```python
from build123d import *

# Parameters (mm, degrees)
BOSS_EXTRUDE1_DEPTH = 4
SKETCH3_R           = 4
SKETCH3_R_2         = 1.5
CUT_EXTRUDE1_DEPTH  = 119.072218241
SKETCH5_R           = 1.5
CUT_EXTRUDE2_DEPTH  = 119.072218241
SKETCH6_R           = 1.5
CUT_EXTRUDE3_DEPTH  = 119.072218241


with BuildPart() as part:
    # Sketch1 → Boss-Extrude1 (new body)
    with BuildSketch(Plane(origin=(0, 0, 0), x_dir=(1, 0, 0), z_dir=(0, 1, 0))):
        Polygon((-55, 61.024984395), (-35, 42), (35, 42), (55, 61.024984395), (81, 61.024984395), (101, 40), (101, -40), (81, -61.024984395), (55, -61.024984395), (35, -42), (-35, -42), (-55, -61.024984395), (-81, -61.024984395), (-101, -40), (-101, 40), (-81, 61.024984395), align=None)
    extrude(amount=BOSS_EXTRUDE1_DEPTH)

    # Sketch3 → Cut-Extrude1 (cut, through all)
    with BuildSketch(Plane(origin=(0, 4, 0), x_dir=(1, 0, 0), z_dir=(0, 1, 0))):
        with Locations(Location((-35, -29, 0), (0, 0, 270))):
            Circle(SKETCH3_R)
        with Locations(Location((-28.5, -29, 0), (0, 0, 270))):
            Circle(SKETCH3_R_2)
        with Locations(Location((-41.5, -29, 0), (0, 0, 270))):
            Circle(SKETCH3_R_2)
        with Locations(Location((-35, -22.5, 0), (0, 0, 270))):
            Circle(SKETCH3_R_2)
        with Locations(Location((-35, -35.5, 0), (0, 0, 270))):
            Circle(SKETCH3_R_2)
        with Locations(Location((-35, 35.5, 0), (0, 0, 90))):
            Circle(SKETCH3_R_2)
        with Locations(Location((-35, 22.5, 0), (0, 0, 90))):
            Circle(SKETCH3_R_2)
        with Locations(Location((-41.5, 29, 0), (0, 0, 90))):
            Circle(SKETCH3_R_2)
        with Locations(Location((-28.5, 29, 0), (0, 0, 90))):
            Circle(SKETCH3_R_2)
        with Locations(Location((-35, 29, 0), (0, 0, 90))):
            Circle(SKETCH3_R)
        with Locations(Location((-35, 0, 0), (0, 0, 270))):
            Circle(SKETCH3_R)
        with Locations(Location((-35, 6.5, 0), (0, 0, 270))):
            Circle(SKETCH3_R_2)
        with Locations(Location((-28.5, 0, 0), (0, 0, 270))):
            Circle(SKETCH3_R_2)
        with Locations(Location((-41.5, 0, 0), (0, 0, 270))):
            Circle(SKETCH3_R_2)
        with Locations(Location((-35, -6.5, 0), (0, 0, 270))):
            Circle(SKETCH3_R_2)
    extrude(amount=-CUT_EXTRUDE1_DEPTH, mode=Mode.SUBTRACT)

    # Sketch5 → Cut-Extrude2 (cut, through all)
    with BuildSketch(Plane(origin=(0, 4, 0), x_dir=(1, 0, 0), z_dir=(0, 1, 0))):
        with Locations(Location((93, 35, 0), (0, 0, 270))):
            Circle(SKETCH5_R)
        with Locations(Location((63, 35, 0), (0, 0, 270))):
            Circle(SKETCH5_R)
        with Locations(Location((63, -35, 0), (0, 0, 90))):
            Circle(SKETCH5_R)
        with Locations(Location((93, -35, 0), (0, 0, 90))):
            Circle(SKETCH5_R)
    extrude(amount=-CUT_EXTRUDE2_DEPTH, mode=Mode.SUBTRACT)

    # Sketch6 → Cut-Extrude3 (cut, through all)
    with BuildSketch(Plane.XZ):
        with Locations(Location((71, 20, 0), (0, 0, 270))):
            Circle(SKETCH6_R)
        with Locations(Location((71, -20, 0), (0, 0, 270))):
            Circle(SKETCH6_R)
    extrude(amount=-CUT_EXTRUDE3_DEPTH, mode=Mode.SUBTRACT)


solid = part.part
```
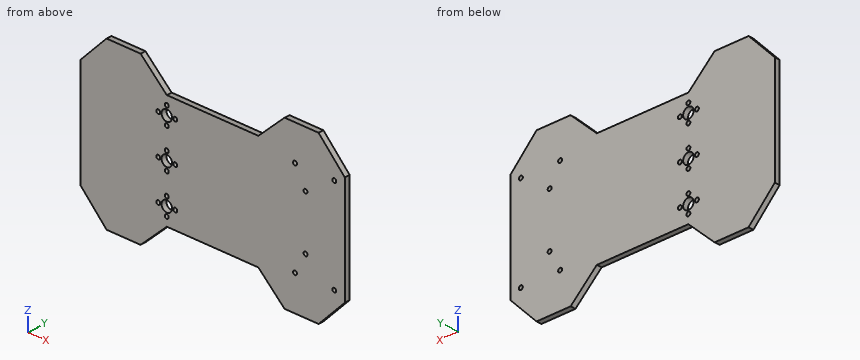
Verification items for the finished model (mm, model axes). Give positions to 0.01 mm unless a question says otherwise; leave off trailing zeros. Order: outer loops, then holes, each group sorted by start corner. A loop starts at its lowest first (then second) coordinate and runs counter-clockwise, first axis right, second up. Notation, with made-up numbers: (21.5, 35.25) - (36.5, 35.25) arc R31 cw to (36.5, 72.25) - close; hole circle Ø1 at (64, 1.5). An arc over 180 degrees is marked (long way). Answer as CSV lines item,"result". Start each with the question number.
Item 1: Section check A-A, the plane z = 46.5. Record the boundary of the cut face in (x, y), plus the area to 3 significant figures.
Item 2: Section check B-B, the plane y = 1.8. State how many separate pieces and enclosed holes the cut face has, plus the area to 3 significant figures.
Item 3: Material ranges on L1, parallel to X at y = 2.9, z = -29; L2, parallel to Z at x = 63.5, y = 0.85; L3, parallel to Z at x = -42, y = 2.9, recorded low to high.
Item 4: Gauge pin test, flat ends, axial feed: pin 1 (2.5 mm diameter, centred on x = -35, z = 22.5, fed in from +Y); pin 2 (2 mm diameter, centred on x = -5, y = 1.5, fed in from +Z). Record the tip position at first contact, or that the pin passes through.
Item 5: Section check C-C, the plane x = 31. Record the boundary of the cut face in (y, z).
Filled in:
1,outline,"(-94.82, 0) - (-39.73, 0) - (-39.73, 4) - (-94.82, 4) - close; (39.73, 0) - (94.82, 0) - (94.82, 4) - (39.73, 4) - close"
1,area,"441 mm^2"
2,separate pieces,"1"
2,enclosed holes,"21"
2,area,"20,100 mm^2"
3,L1,"-101 to -43, -40 to -39, -31 to -30, -27 to 101"
3,L2,"-61.02 to -36.41, -33.59 to 33.59, 36.41 to 61.02"
3,L3,"-48.66 to -30.41, -27.59 to -1.41, 1.41 to 27.59, 30.41 to 48.66"
4,pin 1,"through"
4,pin 2,"z = 42"
5,outline,"(0, -42) - (4, -42) - (4, 42) - (0, 42) - close"
